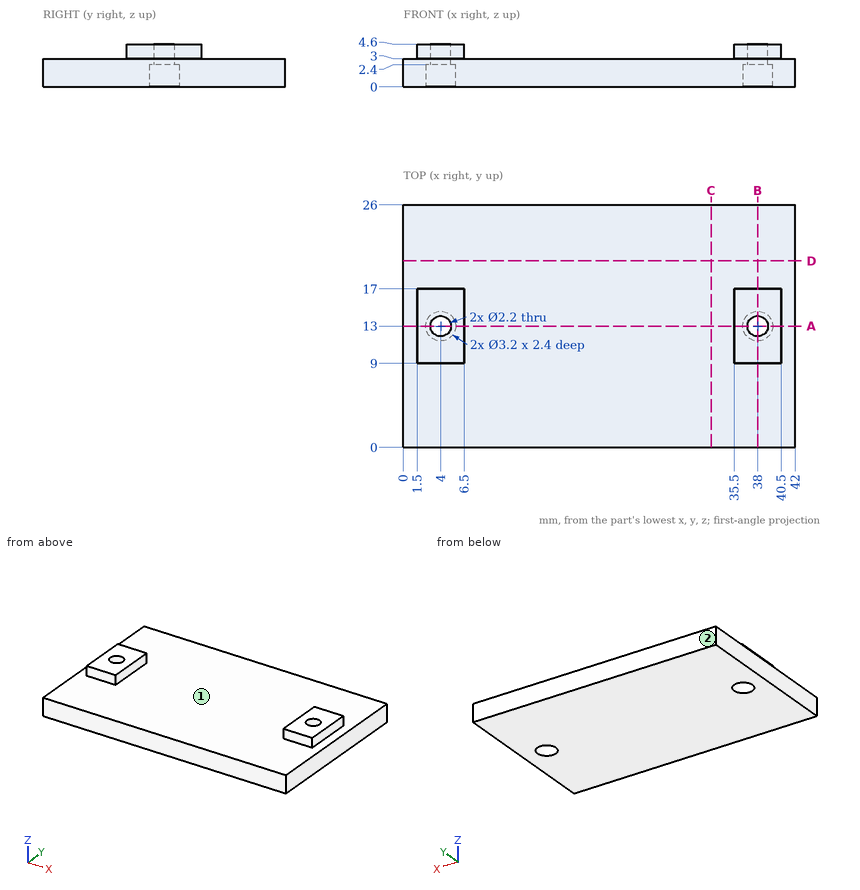
The figure shows three views and two pictorial views of one solid part (mm, origin at its lowest corner). Answer the questions. Round coordinates to 2 decimals unless told otherwise and drop trailing zeros. Order: outer loops, then holes, each group sorted by start corner. A loop starts at its lowest first (then second) coordinate and runs counter-clockwise, first axis right, second up.
Q1. Find the intervals of material crossed by line 1 along X through (y, z) = (13, 3.4); line 2 along Y through (x, z) = (38, 1.25); line 3 along X through (y, z) = (15.5, 3.25), in increasing order.
Solution:
line 1: x = 1.5 to 2.9, 5.1 to 6.5, 35.5 to 36.9, 39.1 to 40.5
line 2: y = 0 to 11.4, 14.6 to 26
line 3: x = 1.5 to 6.5, 35.5 to 40.5
Q2. A cutting plane is placed at C-C, the plane x = 33. Determine the outline of the cut face in (y, z).
Solution:
outline: (0, 0) - (26, 0) - (26, 3) - (0, 3) - close
Q3. A cutting plane is placed at A-A, the plane y = 13. Determine the outline of the cut face in (x, z), then the cut area to 3 significant figures.
Solution:
outline: (0, 0) - (2.4, 0) - (2.4, 2.4) - (2.9, 2.4) - (2.9, 4.6) - (1.5, 4.6) - (1.5, 3) - (0, 3) - close; (5.1, 2.4) - (5.6, 2.4) - (5.6, 0) - (36.4, 0) - (36.4, 2.4) - (36.9, 2.4) - (36.9, 4.6) - (35.5, 4.6) - (35.5, 3) - (6.5, 3) - (6.5, 4.6) - (5.1, 4.6) - close; (39.1, 2.4) - (39.6, 2.4) - (39.6, 0) - (42, 0) - (42, 3) - (40.5, 3) - (40.5, 4.6) - (39.1, 4.6) - close
area: 117 mm2
Q4. Given pin 1 Ø1.8 at (y, z) = (12, 3.5) entering from +X; pin 2 Ø3 at (x, y) = (38, 13) entering from -Z; pin 3 Ø10 at (x, y) = (22.5, 4.5) entering from +Z; pin 4 Ø0.8 at (y, z) = (12, 3.5) entering from -X, each flat-ended and moving along its own axis, determine where each tip first touches the part or whether it passes through.
Solution:
pin 1: stops at x = 42
pin 2: stops at z = 2.4
pin 3: stops at z = 3
pin 4: stops at x = 1.5
Q5. The mould has two halves that part along X. Classify the marked faces 1 and 2: pulls with the +X half, pulls with the -X half, needs draft (parallel to the pull), parting line crosses it, or undercut.
Solution:
face 1: undercut
face 2: needs draft
Q6. A cutting plane is placed at B-B, the plane x = 38. Determine the outline of the cut face in (y, z).
Solution:
outline: (0, 0) - (11.4, 0) - (11.4, 2.4) - (11.9, 2.4) - (11.9, 4.6) - (9, 4.6) - (9, 3) - (0, 3) - close; (14.1, 2.4) - (14.6, 2.4) - (14.6, 0) - (26, 0) - (26, 3) - (17, 3) - (17, 4.6) - (14.1, 4.6) - close
Q7. A cutting plane is placed at D-D, the plane y = 20. Determine the outline of the cut face in (x, z).
Solution:
outline: (0, 0) - (42, 0) - (42, 3) - (0, 3) - close
